Autodesk Fusion 360 part; units mm, degrees
sketch "Sketch1" plane through (0, 0, 0) normal (0, 1, 0) x (1, 0, 0)
  line L0 (0, 0) -> (60, 0)
  line L1 (60, 0) -> (60, -30)
  line L2 (60, -30) -> (0, -30)
  line L3 (0, -30) -> (0, 0)
  line L4 (0, -15) -> (60, -15) construction
  line L5 (8, 0) -> (8, -30) construction
  line L6 (24, 0) -> (24, -30) construction
  line L7 (11, -13) -> (5, -13)
  arc A0 (5, -13) -> (5, -17) centre (5, -15) ccw
  line L8 (5, -17) -> (11, -17)
  arc A1 (11, -17) -> (11, -13) centre (11, -15) ccw
  line L9 (11, -15) -> (5, -15) construction
  line L10 (21, -17) -> (27, -17)
  arc A2 (27, -17) -> (27, -13) centre (27, -15) ccw
  line L11 (27, -13) -> (21, -13)
  arc A3 (21, -13) -> (21, -17) centre (21, -15) ccw
  line L12 (21, -15) -> (27, -15) construction
  line L13 (43, 0) -> (43, -30) construction
  point P0 (11, -15)
  point P1 (5, -15)
  point P2 (21, -15)
  point P3 (27, -15)
  dimension "d1" = 60
  dimension "d2" = 30
  dimension "d3" = 8
  dimension "d4" = 16
  dimension "d5" = 3
  dimension "d6" = 3
  dimension "d7" = 3
  dimension "d8" = 3
  dimension "d9" = 4
  dimension "d10" = 4
  dimension "d13" = 43
extrude "Extrude1" add sketch "Sketch1" along normal blind 9.6
sketch "Sketch2" plane through (0, 9.6, 0) normal (0, 1, 0) x (-1, 0, 0)
  arc A0 (-21, 13) -> (-21, 17) centre (-21, 15) ccw
  line L0 (-21, 13) -> (-27, 13)
  arc A1 (-27, 17) -> (-27, 13) centre (-27, 15) ccw
  line L1 (-27, 17) -> (-21, 17)
  arc A2 (-11, 17) -> (-11, 13) centre (-11, 15) ccw
  line L2 (-11, 17) -> (-5, 17)
  arc A3 (-5, 13) -> (-5, 17) centre (-5, 15) ccw
  line L3 (-5, 13) -> (-11, 13)
  line L4 (0, 30) -> (-60, 30)
  line L5 (-60, 30) -> (-60, 0)
  line L6 (-60, 0) -> (0, 0)
  line L7 (0, 0) -> (0, 30)
  circle A4 centre (-43, 15) radius 11.05
  circle A5 centre (-43, 15) radius 10.55
  dimension "d15" = 22.1
  dimension "d16" = 21.1
extrude "Extrude2" cut sketch "Sketch2" against normal blind 7 contours A4
extrude "Extrude3" cut 1 faces at (40.0944, 9.6, 14.0673) along direction (0, 1, 0) through all and the other way through all
sketch "Sketch3" plane through (0, 9.6, 0) normal (0, 1, 0) x (-1, 0, 0)
  line L0 (0, 30) -> (-60, 30)
  line L1 (-60, 30) -> (-60, 0)
  line L2 (-60, 0) -> (0, 0)
  line L3 (0, 0) -> (0, 30)
  arc A0 (-21, 13) -> (-21, 17) centre (-21, 15) ccw
  line L4 (-21, 13) -> (-27, 13)
  arc A1 (-27, 17) -> (-27, 13) centre (-27, 15) ccw
  line L5 (-27, 17) -> (-21, 17)
  arc A2 (-11, 17) -> (-11, 13) centre (-11, 15) ccw
  line L6 (-11, 17) -> (-5, 17)
  arc A3 (-5, 13) -> (-5, 17) centre (-5, 15) ccw
  line L7 (-5, 13) -> (-11, 13)
  circle A4 centre (-43, 15) radius 11.05
  circle A5 centre (-43, 15) radius 13 construction
  point P0 (-32.8444, 6.8844)
  point P1 (-52.1828, 24.202)
  point P2 (-53.1556, 6.8844)
  dimension "d30" = 26
hole "Hole1" at (32.8444, 9.6, 6.8844) direction (0, -1, 0) diameter 2.5 end through all
hole "Hole2" at (53.1556, 9.6, 6.8844) direction (0, -1, 0) diameter 2.5 end through all
hole "Hole3" at (52.1828, 9.6, 24.202) direction (0, -1, 0) diameter 2.5 end through all
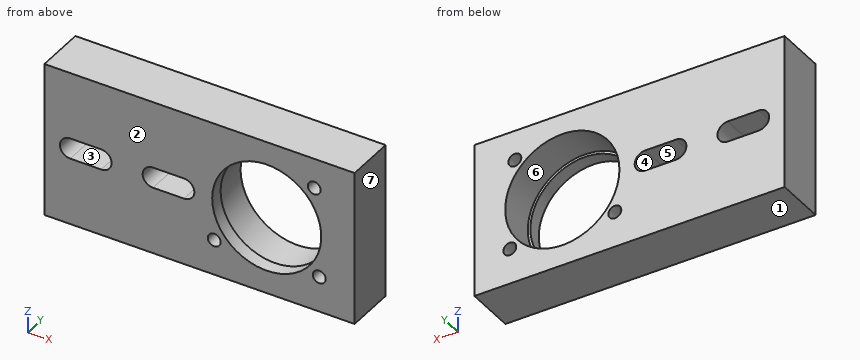
The listing builds one solid part. Answer for the finished solid, in the listing's coordinates (mm). Face numbers are marked on the shaded views. A direction names the side the tool comes from. Round coordinates to 2 decimals unless told otherwise and drop trailing zeros. Loops run counter-clockwise (first coordinate to the right, second up) from the corner with the lowest first, then second, coordinate; pieces in that order, holes last. Notation, with made-up numbers: M 23.25,86.5 L 48.25,86.5 A23 ccw 48.25,113.5 Z; hole C 81.5,-31.75 d1. An arc over 180 degrees is marked long. Write each question's results on one line, items separated by ' | '. Start each with the question number.
1) Find section B-B on x = 43. Write down the section's boundary in (y, z).
2) Find section A-A on z = 15. Write down the section's boundary in (x, y).
3) Determine the mould class of the marked faces 1, 2, 3 and 4 for opening direction Z: pulls with the +Z half, pulls with the -Z half, needs draft (parallel to the pull), parting line crosses it, or undercut.
4) Straight lines are drawn through the part: probe 1 along X at (y, z) = (4.25, 15.25); probe 2 along Z at (x, y) = (40, 4); probe 3 along X at (y, z) = (9, 20). For each, find the intervals that lie inside material, in ascending order.
5) Which of the six approach directions +Z, -Z, +X, -X, +Y, -Y give full straight-line access (tool end or side, diameter ignored) to the marked faces 5, 6 and 7?
6) Find section C-C on y = 1.25. Write down the section's boundary in (x, z).
7) Find section D-D on z = 20.25. Write down the section's boundary in (x, y).
Final values:
1) outline: M 0,0 L 9.6,0 L 9.6,3.95 L 2.6,3.95 L 2.6,4.45 L 0,4.45 Z; M 0,25.55 L 2.6,25.55 L 2.6,26.05 L 9.6,26.05 L 9.6,30 L 0,30 Z
2) outline: M 0,0 L 3,0 L 3,9.6 L 0,9.6 Z; M 13,0 L 19,0 L 19,9.6 L 13,9.6 Z; M 29,0 L 32.45,0 L 32.45,2.6 L 31.95,2.6 L 31.95,9.6 L 29,9.6 Z; M 53.55,0 L 60,0 L 60,9.6 L 54.05,9.6 L 54.05,2.6 L 53.55,2.6 Z
3) face 1: pulls with the -Z half | face 2: needs draft | face 3: undercut | face 4: undercut
4) probe 1: 0 to 3.02, 12.98 to 19.02, 28.98 to 31.95, 54.05 to 60 | probe 2: 0 to 4.37, 25.63 to 30 | probe 3: 0 to 33.15, 52.85 to 60
5) face 5: +Y, -Y | face 6: +Y | face 7: +Z, -Z, +X, +Y, -Y
6) outline: M 0,0 L 60,0 L 60,30 L 0,30 Z; hole M 5,13 L 11,13 A2 ccw 11,17 L 5,17 A2 ccw Z; hole M 21,13 L 27,13 A2 ccw 27,17 L 21,17 A2 ccw Z; hole C 32.84,6.88 d2.5; hole C 43,15 d21.1; hole C 52.18,24.2 d2.5; hole C 53.16,6.88 d2.5
7) outline: M 0,0 L 33.85,0 L 33.85,2.6 L 33.28,2.6 L 33.28,9.6 L 0,9.6 Z; M 52.15,0 L 60,0 L 60,9.6 L 52.72,9.6 L 52.72,2.6 L 52.15,2.6 Z
